Work out the finished part from the listing and answer in its coordinate system (mm). Face numbers are marked on the shaded views. A direction names the side the tool comes from. Round coordinates to 2 decimals unless told otherwise and drop trailing zeros. Loops run counter-clockwise (first coordinate to the right, second up) from the corner with the lowest first, then second, coordinate; pieces in that order, holes last. Notation, with made-up numbers: (-28, 68) - (6, 68) arc R28 ccw to (6, 97) - close; hole circle Ø8 at (-29, -7). An arc over 180 degrees is marked (long way). Answer as CSV lines item,"result". Start each with the question number.
Q1. Section A-A on z = 20 is taken. Write down the section's boundary in (x, y), then the cut area to 3 significant figures.
Q2. Straight lines are drawn through the part: L1, parallel to X at y = 29, z = 75; L2, parallel to Z at x = 32.5, y = -30; L3, parallel to X at y = 55.5, z = 66. For each, find the intervals that lie inside material, in ascending order. Write a range as [from, to].
Q3. The mould has two halves that part along Z. Classify the marked faces 6, 7, 8 and 9: +Z half, -Z half, draft (parallel to the pull), parting line (faces both ways), or undercut.
Q4. For the marked faces 1, 2, 3, 4 and 5, determine the directions among +Z, -Z, +X, -X, +Y, -Y from which every point of the face is accessible in a straight line to the end or side of a thin tool.
Q5. Section D-D on z = 103 is taken. Write down the section's boundary in (x, y).
Q6. Section B-B on x = 112.5 is taken. Write down the section's boundary in (y, z), then the cut area to 3 significant figures.
Q7. Each of these flat-tipped pins is pushed along its axis until it touches: pin 1 Ø10 at (x, z) = (-34, 162.5) entering from -Y; pin 2 Ø11.5 at (x, y) = (51.27, -51.27) entering from -Z; pin 3 Ø14.5 at (x, y) = (-51.27, -51.27) entering from +Z; pin 4 Ø16.5 at (x, z) = (54, 92) entering from +Y. Where does it stop, or does it pass through?
Q8. Section C-C on x = 0 is taken. Write down the section's boundary in (y, z).
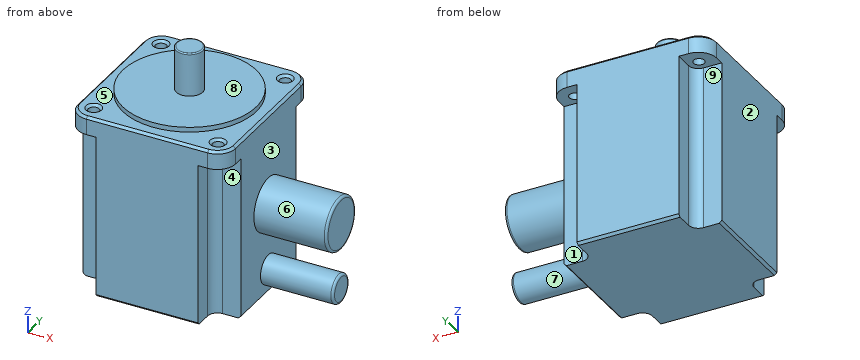
```python
from build123d import *

# Parameters (mm, degrees)
PAD_DEPTH            = 150
SKETCH001_R          = 11
PAD001_DEPTH         = 40
FILLET_R             = 1
SKETCH002_R          = 22
SKETCH002_R_2        = 12
PAD002_DEPTH         = 60
SKETCH003_R          = 4.5
POCKET_DEPTH         = 25
FILLET001_R          = 2
CHAMFER_SIZE         = 2
SKETCH004_R          = 55
PAD003_DEPTH         = 4
POCKET001_DEPTH      = 135
BODY_PLACEMENT_ANGLE = 180


with BuildPart() as part:
    # Sketch → Pad (new body)
    with BuildSketch(Plane.XY):
        with BuildLine():
            Line((-50, 65), (50, 65))
            ThreePointArc((65, 50), (60.606602, 60.606602), (50, 65))
            Line((65, 50), (65, -50))
            ThreePointArc((50, -65), (60.606602, -60.606602), (65, -50))
            Line((50, -65), (-50, -65))
            ThreePointArc((-65, -50), (-60.606602, -60.606602), (-50, -65))
            Line((-65, -50), (-65, 50))
            ThreePointArc((-50, 65), (-60.606602, 60.606602), (-65, 50))
        make_face()
    extrude(amount=PAD_DEPTH)

    # Sketch001 (on Face10 of Pad) → Pad001 (join)
    with BuildSketch(Plane.XY.offset(150)):
        Circle(SKETCH001_R)
    extrude(amount=PAD001_DEPTH)

    # Fillet
    fillet_edges = [part.edges().sort_by_distance(p)[0] for p in [
        (-11, 0, 190),
    ]]
    fillet(fillet_edges, radius=FILLET_R)

    # Sketch002 (on Face8 of Fillet) → Pad002 (join)
    with BuildSketch(Plane(origin=(-65, 0, 0), x_dir=(0, -1, 0), z_dir=(-1, 0, 0))):
        with Locations((0, 75)):
            Circle(SKETCH002_R)
        with Locations((0, 20)):
            Circle(SKETCH002_R_2)
    extrude(amount=PAD002_DEPTH)

    # Sketch003 (on Face3 of Pad002) → Pocket (cut)
    with BuildSketch(Plane.XY.offset(150)):
        with Locations((-51.265242, 51.265242)):
            Circle(SKETCH003_R)
        with Locations((51.265242, 51.265242)):
            Circle(SKETCH003_R)
        with Locations((51.265242, -51.265242)):
            Circle(SKETCH003_R)
        with Locations((-51.265242, -51.265242)):
            Circle(SKETCH003_R)
    extrude(amount=-POCKET_DEPTH, mode=Mode.SUBTRACT)

    # Fillet001
    fillet001_edges = [part.edges().sort_by_distance(p)[0] for p in [
        (-125, 12, 20),
        (-125, 22, 75),
    ]]
    fillet(fillet001_edges, radius=FILLET001_R)

    # Chamfer
    chamfer_edges = [part.edges().sort_by_distance(p)[0] for p in [
        (-65, 0, 150),
        (0, 65, 150),
        (65, 0, 150),
        (0, -65, 150),
        (60.606602, -60.606602, 150),
        (-60.606602, -60.606602, 150),
        (-60.606602, 60.606602, 150),
        (60.606602, 60.606602, 150),
        (-55.765242, -51.265242, 150),
        (46.765242, -51.265242, 150),
        (-55.765242, 51.265242, 150),
        (-11, 0, 150),
        (46.765242, 51.265242, 150),
        (-65, 0, 0),
        (-60.606602, 60.606602, 0),
        (-60.606602, -60.606602, 0),
        (0, 65, 0),
        (60.606602, 60.606602, 0),
        (65, 0, 0),
        (60.606602, -60.606602, 0),
        (0, -65, 0),
    ]]
    chamfer(chamfer_edges, length=CHAMFER_SIZE)

    # Sketch004 (on Face13 of Chamfer) → Pad003 (join)
    with BuildSketch(Plane.XY.offset(150)):
        Circle(SKETCH004_R)
    extrude(amount=PAD003_DEPTH)

    # Sketch005 (on Face11 of Pad003) → Pocket001 (cut)
    with BuildSketch(Plane(origin=(0, 0, 0), x_dir=(1, 0, 0), z_dir=(0, 0, -1))):
        with BuildLine():
            ThreePointArc((-42, -50), (-44.343146, -44.343146), (-50, -42))
            Line((-50, -42), (-65, -42))
            Line((-65, -50), (-65, -42))
            ThreePointArc((-65, -50), (-60.606602, -60.606602), (-50, -65))
            Line((-50, -65), (-42, -65))
            Line((-42, -50), (-42, -65))
        make_face()
        with BuildLine():
            ThreePointArc((50, -42), (44.343146, -44.343146), (42, -50))
            Line((42, -50), (42, -65))
            Line((50, -65), (42, -65))
            ThreePointArc((50, -65), (60.606602, -60.606602), (65, -50))
            Line((65, -50), (65, -42))
            Line((50, -42), (65, -42))
        make_face()
        with BuildLine():
            ThreePointArc((-50, 42), (-44.343146, 44.343146), (-42, 50))
            Line((-42, 50), (-42, 65))
            Line((-50, 65), (-42, 65))
            ThreePointArc((-50, 65), (-60.606602, 60.606602), (-65, 50))
            Line((-65, 50), (-65, 42))
            Line((-50, 42), (-65, 42))
        make_face()
        with BuildLine():
            ThreePointArc((42, 50), (44.343146, 44.343146), (50, 42))
            Line((50, 42), (65, 42))
            Line((65, 50), (65, 42))
            ThreePointArc((65, 50), (60.606602, 60.606602), (50, 65))
            Line((50, 65), (42, 65))
            Line((42, 50), (42, 65))
        make_face()
    extrude(amount=-POCKET001_DEPTH, mode=Mode.SUBTRACT)


with BuildPart() as part_1:
    # Body placement: moved
    add(part.part.rotate(Axis((0, 0, 0), (0, 0, 1)), BODY_PLACEMENT_ANGLE))


solid = part_1.part
```
Findings:
1,outline,"(-65, -42) - (-50, -42) arc R8 cw to (-42, -50) - (-42, -65) - (42, -65) - (42, -50) arc R8 cw to (50, -42) - (65, -42) - (65, -12) - (123, -12) arc R2 ccw to (125, -10) - (125, 10) arc R2 ccw to (123, 12) - (65, 12) - (65, 42) - (50, 42) arc R8 cw to (42, 50) - (42, 65) - (-42, 65) - (-42, 50) arc R8 cw to (-50, 42) - (-65, 42) - close"
1,area,"16,300 mm^2"
2,L1,"x = [-65, 65]"
2,L2,"z = [0, 154]"
2,L3,"x = [-42, 42]"
3,face 6,"undercut"
3,face 7,"undercut"
3,face 8,"+Z half"
3,face 9,"draft"
4,face 1,"-Z, +X, +Y"
4,face 2,"+Z, -Z, -X, +Y, -Y"
4,face 3,"+X"
4,face 4,"-Z, +X, -Y"
4,face 5,"+Z"
5,outline,"(-65, -42) - (-50, -42) arc R8 cw to (-42, -50) - (-42, -65) - (42, -65) - (42, -50) arc R8 cw to (50, -42) - (65, -42) - (65, 42) - (50, 42) arc R8 cw to (42, 50) - (42, 65) - (-42, 65) - (-42, 50) arc R8 cw to (-50, 42) - (-65, 42) - close"
6,outline,"circle Ø44 at (0, 75); circle Ø24 at (0, 20)"
6,area,"1,970 mm^2"
7,pin 1,"passes through"
7,pin 2,"stops at z = 135"
7,pin 3,"stops at z = 150"
7,pin 4,"stops at y = 43.22"
8,outline,"(-65, 2) - (-63, 0) - (63, 0) - (65, 2) - (65, 148) - (63, 150) - (55, 150) - (55, 154) - (11, 154) - (11, 189) arc R1 ccw to (10, 190) - (-10, 190) arc R1 ccw to (-11, 189) - (-11, 154) - (-55, 154) - (-55, 150) - (-63, 150) - (-65, 148) - close"
